Here's the drawing with two shaded views (mm, measured from the low corner). I have some questions. Give positions to 0.01 mm unless a question says otherwise; leave off trailing zeros. Loops run counter-clockwise (first coordinate to the right, second up) from the corner with the lowest first, then second, coordinate; pieces in that order, holes last.
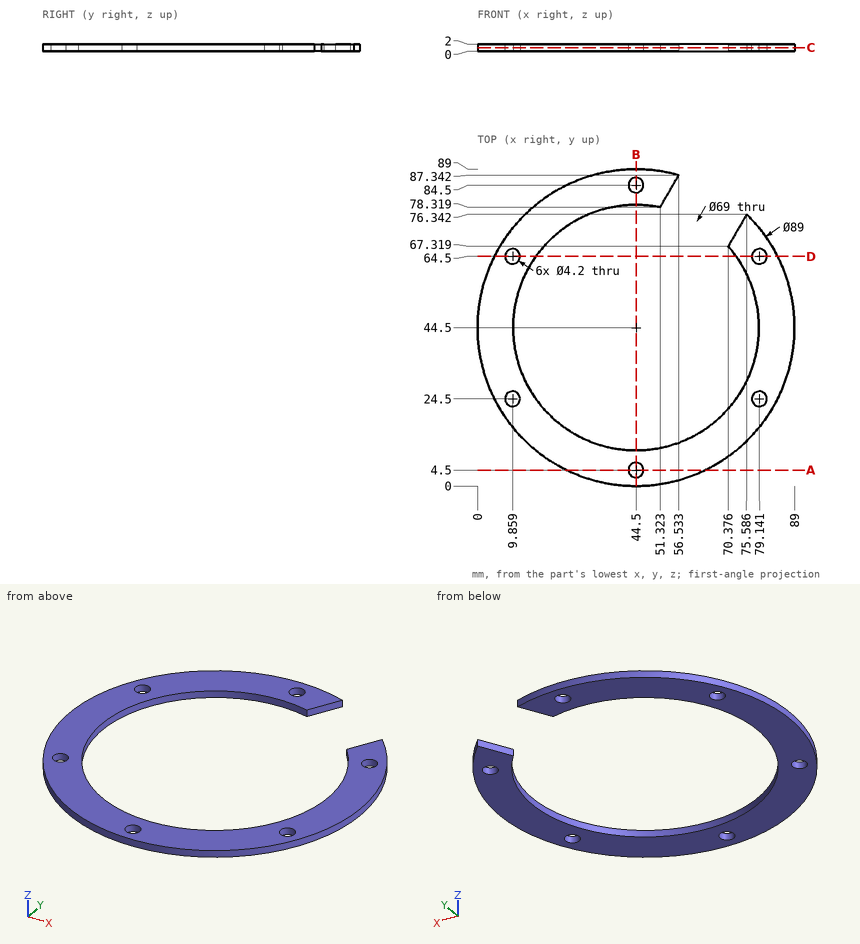
(1) Suppose I cut it at A-A on y = 4.5. List the corners of the cut face in (x, z) for me.
Returned:
outline: (25, 0) - (42.4, 0) - (42.4, 2) - (25, 2) - close; (46.6, 0) - (64, 0) - (64, 2) - (46.6, 2) - close
(2) Suppose I cut it at C-C on z = 0.95. List the corners of the cut face in (x, y) for me (1 decimal), plus the area to 3 significant figures.
Returned:
outline: (51.3, 78.3) - (56.5, 87.3) arc R44.5 ccw (long way) to (75.6, 76.3) - (70.4, 67.3) arc R34.5 cw (long way) to start; hole circle Ø4.2 at (9.9, 24.5); hole circle Ø4.2 at (9.9, 64.5); hole circle Ø4.2 at (44.5, 4.5); hole circle Ø4.2 at (44.5, 84.5); hole circle Ø4.2 at (79.1, 24.5); hole circle Ø4.2 at (79.1, 64.5)
area: 2,180 mm2
(3) Please list where these lines run through material, in increasing order: probe 1 along Y at (x, z) = (44.5, 0.7); probe 2 along Y at (x, z) = (43.5, 0.3) (1 decimal); probe 3 along Y at (x, z) = (41, 1).
Returned:
probe 1: y = 0 to 2.4, 6.6 to 10, 79 to 82.4, 86.6 to 89
probe 2: y = 0 to 2.7, 6.3 to 10, 79 to 82.7, 86.3 to 89
probe 3: y = 0.14 to 10.18, 78.82 to 88.86
(4) Will this pin go through, and if not, where does the flat tip stop? P1, Ø3.5, axis at x = 79.14, y = 64.5, coming from the -Z side.
Returned:
P1: passes through
(5) Suppose I cut it at D-D on y = 64.5. List the corners of the cut face in (x, z) for me.
Returned:
outline: (4.75, 0) - (7.76, 0) - (7.76, 2) - (4.75, 2) - close; (11.96, 0) - (16.39, 0) - (16.39, 2) - (11.96, 2) - close; (72.61, 0) - (77.04, 0) - (77.04, 2) - (72.61, 2) - close; (81.24, 0) - (84.25, 0) - (84.25, 2) - (81.24, 2) - close
(6) Suppose I cut it at B-B on x = 44.5. List the corners of the cut face in (y, z) for me.
Returned:
outline: (0, 0) - (2.4, 0) - (2.4, 2) - (0, 2) - close; (6.6, 0) - (10, 0) - (10, 2) - (6.6, 2) - close; (79, 0) - (82.4, 0) - (82.4, 2) - (79, 2) - close; (86.6, 0) - (89, 0) - (89, 2) - (86.6, 2) - close
